from build123d import *

# Parameters (mm, degrees)
SKETCH_2_W          = 35
SKETCH_2_H          = 36
SKETCH_2_R          = 1.3
SKETCH_2_R_2        = 6.5
EXTRUDE_1_DEPTH     = 3
SKETCH_4_W          = 5
SKETCH_4_H          = 36
EXTRUDE_2_DEPTH     = 20
FILLET_1_R          = 2
CUT_EXTRUDE_1_DEPTH = 2.5
SKETCH_7_R          = 1.6
CUT_EXTRUDE_2_DEPTH = 10


with BuildPart() as part:
    # ｽｹｯﾁ2 → ﾎﾞｽ - 押し出し1 (new body)
    with BuildSketch(Plane(origin=(0, 0, 0), x_dir=(0, 0, -1), z_dir=(1, 0, 0))):
        Rectangle(SKETCH_2_W, SKETCH_2_H)
        with Locations((-14.5, 6)):
            Circle(SKETCH_2_R, mode=Mode.SUBTRACT)
        with Locations((6.5, 6)):
            Circle(SKETCH_2_R, mode=Mode.SUBTRACT)
        with Locations((-14.5, -15)):
            Circle(SKETCH_2_R, mode=Mode.SUBTRACT)
        with Locations((6.5, -15)):
            Circle(SKETCH_2_R, mode=Mode.SUBTRACT)
        with Locations((-4, 6)):
            Circle(SKETCH_2_R_2, mode=Mode.SUBTRACT)
    extrude(amount=EXTRUDE_1_DEPTH)

    # ｽｹｯﾁ4 → ﾎﾞｽ - 押し出し2 (add)
    with BuildSketch(Plane.ZY):
        with Locations((-15, 0)):
            Rectangle(SKETCH_4_W, SKETCH_4_H)
    extrude(amount=EXTRUDE_2_DEPTH)

    # ﾌｨﾚｯﾄ1
    fillet_1_edges = [part.edges().sort_by_distance(p)[0] for p in [
        (0, 0, -12.5),
    ]]
    fillet(fillet_1_edges, radius=FILLET_1_R)

    # ｽｹｯﾁ5 → ｶｯﾄ - 押し出し1 (cut)
    with BuildSketch(Plane.XY.offset(-12.5)):
        Polygon((-12.882308546, 14), (-14.441154273, 16.7), (-17.558845727, 16.7), (-19.117691454, 14), (-17.558845727, 11.3), (-14.441154273, 11.3), align=None)
        Polygon((-2.882308546, 14), (-4.441154273, 16.7), (-7.558845727, 16.7), (-9.117691454, 14), (-7.558845727, 11.3), (-4.441154273, 11.3), align=None)
        Polygon((-12.882308546, -14), (-14.441154273, -11.3), (-17.558845727, -11.3), (-19.117691454, -14), (-17.558845727, -16.7), (-14.441154273, -16.7), align=None)
        Polygon((-2.882308546, -14), (-4.441154273, -11.3), (-7.558845727, -11.3), (-9.117691454, -14), (-7.558845727, -16.7), (-4.441154273, -16.7), align=None)
    extrude(amount=-CUT_EXTRUDE_1_DEPTH, mode=Mode.SUBTRACT)

    # ｽｹｯﾁ7 → ｶｯﾄ - 押し出し2 (cut)
    with BuildSketch(Plane.XY.offset(-15)):
        with Locations((-16, 14)):
            Circle(SKETCH_7_R)
        with Locations((-6, 14)):
            Circle(SKETCH_7_R)
        with Locations((-16, -14)):
            Circle(SKETCH_7_R)
        with Locations((-6, -14)):
            Circle(SKETCH_7_R)
    extrude(amount=-CUT_EXTRUDE_2_DEPTH, mode=Mode.SUBTRACT)


solid = part.part
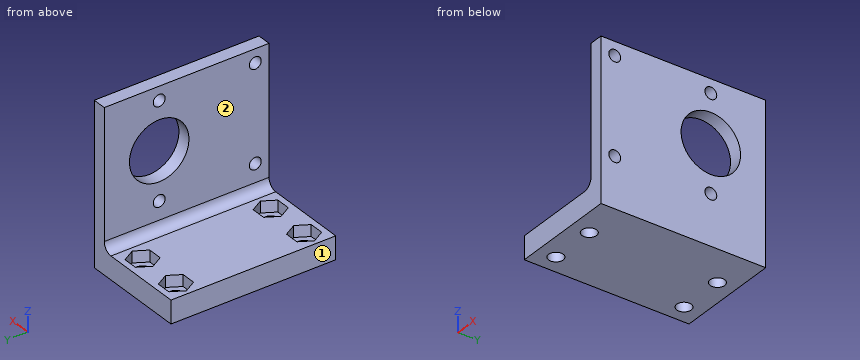
Could you check a few things on this model? Use its own coordinates, in mm. Face numbers are marked on the shaded views. A direction names the side the tool comes from. Give positions to 0.01 mm unless a question says otherwise; leave off trailing zeros. Order: outer loops, then holes, each group sorted by start corner. A loop starts at its lowest first (then second) coordinate and runs counter-clockwise, first axis right, second up.
1. I need wall thicknesses on L1, parallel to Y at x = 2.05, z = 14.5; L2, parallel to Y at x = 1.1, z = 4; L3, parallel to Y at x = -6, z = -15.7. Which ranges of each line are inside material? Lowest first, please.
2. Suppose I cut it at D-D (x = -6). List the corners of the cut face in (y, z) for me.
3. Suppose I cut it at C-C (z = 14.5). List the corners of the cut face in (x, y) for me.
4. Will these pins go through, and if not, where does the flat tip stop? P1, Ø4.5, axis at x = -17, y = 14, coming from the +Z side; P2, Ø5, axis at x = -6, y = -14, coming from the +Z side; P3, Ø3, axis at x = -16, y = -14, coming from the +Z side; P4, Ø10, axis at y = 8.5, z = 2.5, coming from the -X side.
5. Suppose I cut it at A-A (y = 6). List the corners of the cut face in (x, z) for me.
6. Suppose I cut it at B-B (z = 4). List the corners of the cut face in (x, y) for me.
7. For the marked faces 1 and 2, which set-ups out of +Z, -Z, +X, -X, +Y, -Y let a thin tool reach every point of the face, with its end or its side?
Solved:
1. L1: y = -18 to -16.3, -13.7 to 4.7, 7.3 to 18
1. L2: y = -18 to -0.5, 12.5 to 18
1. L3: y = -18 to -15.6, -12.4 to 12.4, 15.6 to 18
2. outline: (-18, -17.5) - (-15.6, -17.5) - (-15.6, -15) - (-16.7, -15) - (-16.7, -12.5) - (-18, -12.5) - close; (-12.4, -17.5) - (12.4, -17.5) - (12.4, -15) - (11.3, -15) - (11.3, -12.5) - (-11.3, -12.5) - (-11.3, -15) - (-12.4, -15) - close; (15.6, -17.5) - (18, -17.5) - (18, -12.5) - (16.7, -12.5) - (16.7, -15) - (15.6, -15) - close
3. outline: (0, -18) - (3, -18) - (3, -16.3) - (0, -16.3) - close; (0, -13.7) - (3, -13.7) - (3, 4.7) - (0, 4.7) - close; (0, 7.3) - (3, 7.3) - (3, 18) - (0, 18) - close
4. P1: stops at z = -12.5
4. P2: stops at z = -15
4. P3: passes through
4. P4: stops at x = 0
5. outline: (-20, -17.5) - (3, -17.5) - (3, -7.8) - (0, -7.8) - (0, -10.5) arc R2 cw to (-2, -12.5) - (-20, -12.5) - close; (0, -5.2) - (3, -5.2) - (3, -2.5) - (0, -2.5) - close; (0, 10.5) - (3, 10.5) - (3, 13.2) - (0, 13.2) - close; (0, 15.8) - (3, 15.8) - (3, 17.5) - (0, 17.5) - close
6. outline: (0, -18) - (3, -18) - (3, -0.5) - (0, -0.5) - close; (0, 12.5) - (3, 12.5) - (3, 18) - (0, 18) - close
7. face 1: +Z, -Z, -X, +Y, -Y
7. face 2: +Z, -X, +Y, -Y
